Autodesk Inventor part; units mm, degrees
ref_plane "YZ Plane" through (0, 0, 0) normal (1, 0, 0) x (0, 1, 0)
ref_plane "XZ Plane" through (0, 0, 0) normal (0, 1, 0) x (-1, 0, 0)
ref_plane "XY Plane" through (0, 0, 0) normal (0, 0, 1) x (1, 0, 0)
sketch "Sketch1" plane through (0, 0, 0) normal (0, 0, 1) x (1, 0, 0)
  line L0 (-69.598, 209.799) -> (-69.598, -40.201) construction
  line L1 (-89.598, 209.799) -> (-89.598, -40.201)
  line L2 (-49.598, -40.201) -> (-49.598, 209.799)
  arc A0 (-49.598, 209.799) -> (-89.598, 209.799) centre (-69.598, 209.799) ccw
  arc A1 (-89.598, -40.201) -> (-49.598, -40.201) centre (-69.598, -40.201) ccw
  point P0 (0, 0)
  point P1 (-69.598, 84.799)
  dimension "d0" = 250
  dimension "d1" = 20
extrude "Extrusion1" add sketch "Sketch1" along normal blind 15
sketch "Sketch2" plane through (0, 0, 0) normal (0, 0, -1) x (-1, 0, 0)
  line L0 (49.598, -40.201) -> (49.598, 209.799)
  circle A0 centre (69.598, 208.3571) radius 12.5
  point P0 (0, 0)
  point P1 (69.598, 88.3571)
  dimension "d4" = 20
  dimension "d5" = 25
  dimension "d6" = 120
extrude "Extrusion2" cut sketch "Sketch2" against normal blind 20
sketch "Sketch3" plane through (0, 0, 0) normal (0, 0, -1) x (-1, 0, 0)
  line L0 (89.598, 209.799) -> (89.598, -40.201)
  circle A0 centre (69.598, -35.201) radius 12.5
  point P0 (0, 0)
  point P1 (69.598, 84.799)
  dimension "d9" = 20
  dimension "d10" = 125
  dimension "d11" = 25
  dimension "d12" = 120
  dimension "d13" = 20
extrude "Extrusion3" cut sketch "Sketch3" against normal blind 20
properties part number "drawing bot arm"
Model file for the job. Use its own axes, mm. Coordinates: 2 decimals unless noted, no trailing zeros. Loops run counter-clockwise (first coordinate to the right, second up) from the corner with the lowest first, then second, coordinate; pieces in that order, holes last. Notation, with made-up numbers: (29.25, -23) - (45.25, -23) arc R21 cw to (45.25, 11) - close; hole circle Ø1 at (21, -10). An arc over 180 degrees is marked (long way). Write item = value, one per line. Start each with the question number.
Item 1: Saw through at C-C, the plane x = -75.5. List the corners of the cut face in (y, z), then the cut area to 3 significant figures.
Item 2: Drop flat-ended pins along their axis: pin 1 Ø8 at (x, z) = (-56.5, 6.5) entering from +Y; pin 2 Ø12 at (x, y) = (-64, 115) entering from -Z; pin 3 Ø2 at (x, z) = (-76, 10.5) entering from -Y; pin 4 Ø1.5 at (x, z) = (-73.5, 3) entering from -Y. Give the stop position or say it passes through.
Item 3: Wall check: probe 1 along X at (y, z) = (208, 6.75); probe 2 along Y at (x, z) = (-76.5, 9.75); probe 3 along Y at (x, z) = (-60, 8.25). Give the ranges that are in metal, low to high. Write a range as [from, to].
Item 4: Pull direction Y, two halves, no side cores. Call faces 1 (the face through (-60.385, -26.753, 7.395)), 2 (the face through (-69.158, -60.196, 7.395)), 3 (the face through (-70, 87, 0)), 4 (the face through (-66.888, 196.154, 7.395)): +Y half, -Y half, draft (parallel to the pull), parting line (faces both ways), or undercut.
Item 5: Saw through at D-D, the plane x = -54.5. List the corners of the cut face in (y, z).
Item 6: Saw through at A-A, the plane x = -65. List the corners of the cut face in (y, z).
Item 7: Saw through at B-B, the plane z = 7.25. List the corners of the cut face in (x, y), then the cut area to 3 significant figures.
Answers:
q1.outline = (-59.31, 0) - (-46.22, 0) - (-46.22, 15) - (-59.31, 15) - close; (-24.18, 0) - (197.34, 0) - (197.34, 15) - (-24.18, 15) - close; (219.38, 0) - (228.91, 0) - (228.91, 15) - (219.38, 15) - close
q1.area = 3,660 mm2
q2.pin_1 = 227.61
q2.pin_2 = 0
q2.pin_3 = -59.46
q2.pin_4 = -59.95
q3.probe_1 = [-89.6, -82.09], [-57.1, -49.6]
q3.probe_2 = [-58.97, -45.62], [-24.78, 197.94], [218.78, 228.57]
q3.probe_3 = [-57.75, -43.21], [-27.19, 200.35], [216.37, 227.35]
q4.face_1 = undercut
q4.face_2 = -Y half
q4.face_3 = draft
q4.face_4 = undercut
q5.outline = (-53.32, 0) - (222.92, 0) - (222.92, 15) - (-53.32, 15) - close
q6.outline = (-59.67, 0) - (-46.82, 0) - (-46.82, 15) - (-59.67, 15) - close; (-23.58, 0) - (196.73, 0) - (196.73, 15) - (-23.58, 15) - close; (219.98, 0) - (229.26, 0) - (229.26, 15) - (219.98, 15) - close
q7.outline = (-89.6, -40.2) arc R20 ccw to (-49.6, -40.2) - (-49.6, 209.8) arc R20 ccw to (-89.6, 209.8) - close; hole circle Ø25 at (-69.6, -35.2); hole circle Ø25 at (-69.6, 208.36)
q7.area = 10,300 mm2
